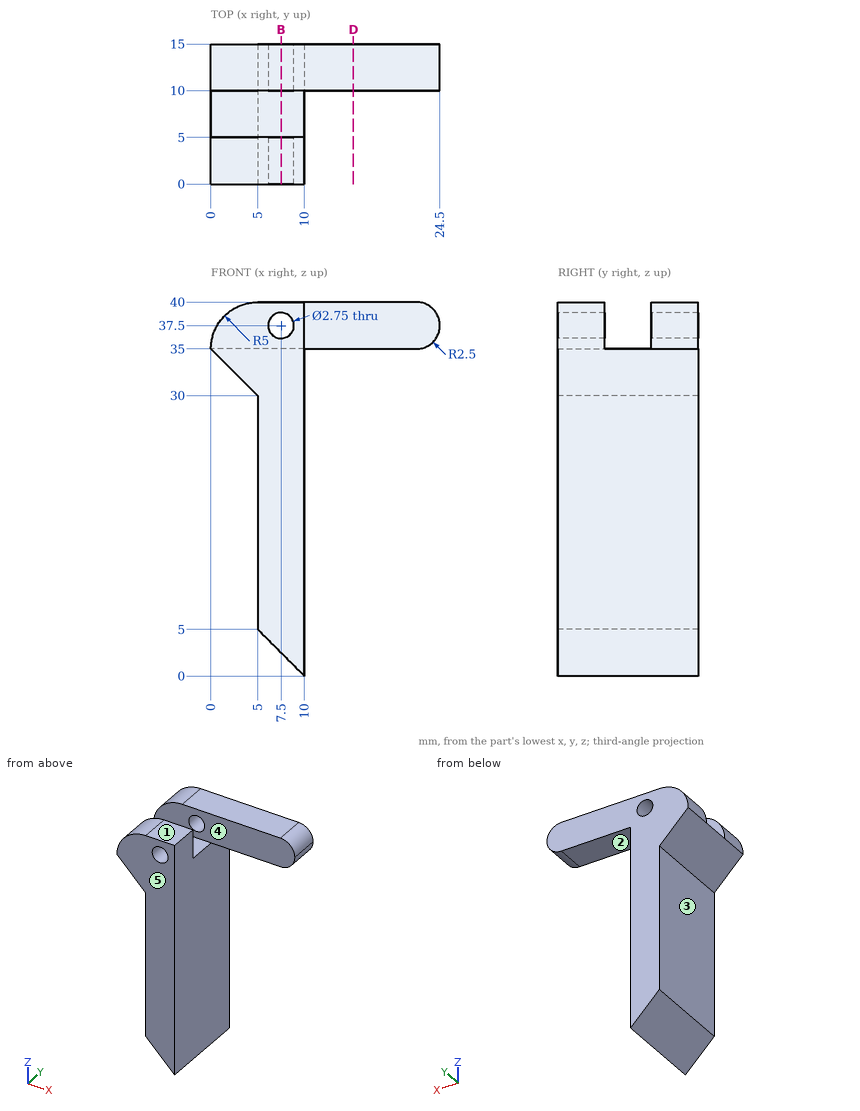
Source: three-view drawing plus pictorial views. Frame: mm from the lowest corner of the part. A direction names the side the tool comes from. Coordinates: 2 decimals unless noted, no trailing zeros. Loops run counter-clockwise (first coordinate to the right, second up) from the corner with the lowest first, then second, coordinate; pieces in that order, holes last. Notation, with made-up numbers: (-16.75, 80) -> (21.25, 80) arc R12 cw to (21.25, 85) -> close; hole circle Ø3 at (53, 46). An arc over 180 degrees is marked (long way). One line per item, written item: value.
(1) Draft query along Y for the marked faces 3, 4 and 5. Return one class per face: pulls with the +Y half, pulls with the -Y half, needs draft (parallel to the pull), parting line crosses it, or undercut.
Answer below:
face 3: needs draft
face 4: undercut
face 5: pulls with the -Y half
(2) Ray query, line 1 along X through (y, z) = (4, 24); line 2 along X through (y, z) = (1.55, 37.5) (3 decimals); line 3 along Z through (x, y) = (7.5, 3.1) (3 decimals). Return the intervals inside material, ascending.
Answer below:
line 1: x = 5 to 10
line 2: x = 0.67 to 6.125, 8.875 to 10
line 3: z = 2.5 to 36.125, 38.875 to 40
(3) Cut plane D-D (x = 15.25). Output: boundary loops of the cut face in (y, z), then the cut area to 3 significant figures.
Answer below:
outline: (10, 35) -> (15, 35) -> (15, 40) -> (10, 40) -> close
area: 25.0 mm2
(4) Cut plane B-B (x = 7.5). Output: boundary loops of the cut face in (y, z) (3 decimals).
Answer below:
outline: (0, 2.5) -> (15, 2.5) -> (15, 36.125) -> (10, 36.125) -> (10, 35) -> (5, 35) -> (5, 36.125) -> (0, 36.125) -> close; (0, 38.875) -> (5, 38.875) -> (5, 40) -> (0, 40) -> close; (10, 38.875) -> (15, 38.875) -> (15, 40) -> (10, 40) -> close
(5) Pin query (flat end, axial travel): pin 1 Ø1.5 at (x, z) = (11, 36.5) entering from -Y; pin 2 Ø3 at (y, z) = (6, 12.5) entering from -X; pin 3 Ø5 at (y, z) = (6.5, 32.5) entering from +X. Return the tip coordinate at first contact, or that it passes through.
Answer below:
pin 1: stops at y = 10
pin 2: stops at x = 5
pin 3: stops at x = 10
(6) Set-up query: the marked faces 1 and 2. Return all of +Z, -Z, +X, -X, +Y, -Y with unobstructed straight access to the full face (end or side cutting, diameter ignored); none if empty.
Answer below:
face 1: +Z, +X, -X, +Y, -Y
face 2: -Z, +X, +Y, -Y
